Can you work these out from the drawing? Everything is in mm from the part's minimum corner. A direction names the side the tool comes from. Round coordinates to 2 decimals unless told otherwise and drop trailing zeros. Order: outer loops, then holes, each group sorted by start corner. A loop starts at its lowest first (then second) coordinate and runs counter-clockwise, first axis right, second up. Notation, with made-up numbers: (1.5, -35.5) -> (40.5, -35.5) arc R21 cw to (40.5, 3.5) -> close; hole circle Ø3 at (20.5, -5). An arc over 180 degrees is marked (long way). Use a Markdown table: item, result. Add a question column.
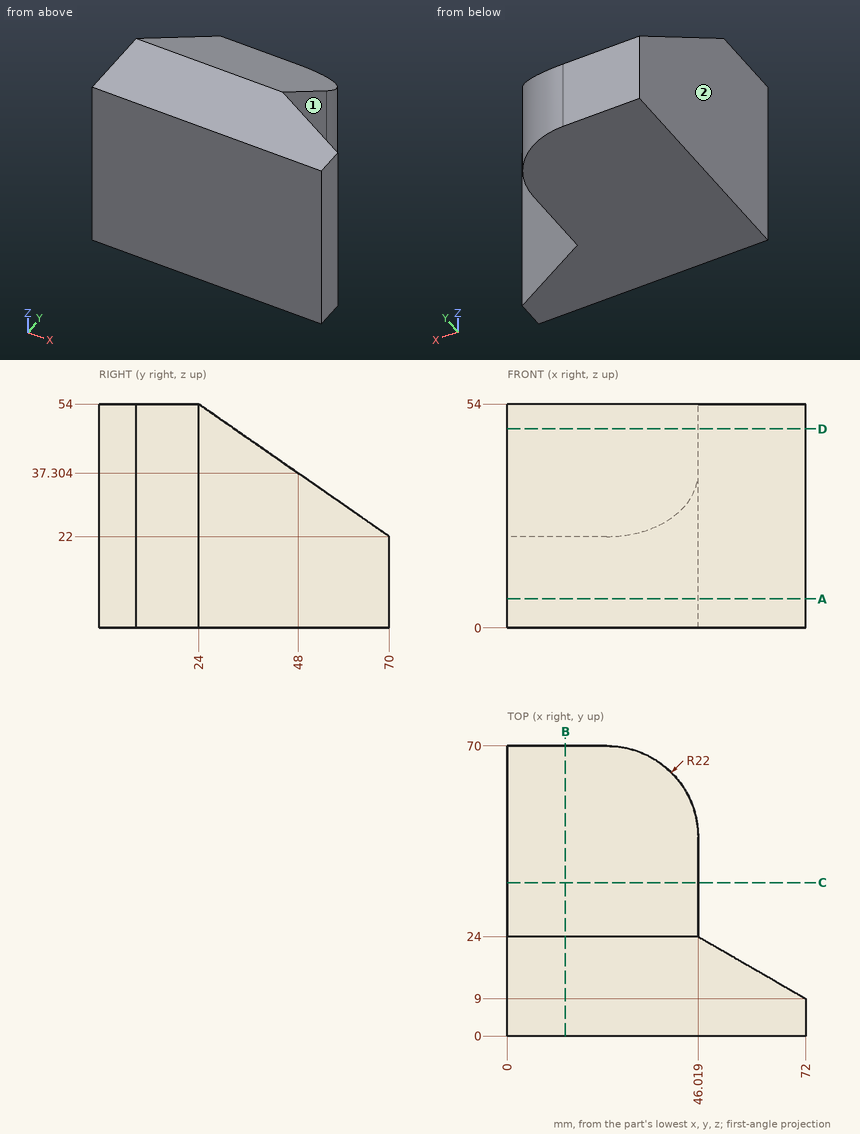
(1) I'm going to push flat-ended pins straight in: P1, Ø12, axis at y = 39, z = 31.5, coming from the +X side; P2, Ø1.5, axis at y = 15.5, z = 20, coming from the +X side; P3, Ø6, axis at x = 16, z = 30.5, coming from the +Y side (1 decimal). Where does each tip first touch, or does it pass through?
(2) Please list where these lines run through material, in increasing order: probe 1 along X at (y, z) = (39.5, 24.5); probe 2 along Z at (x, y) = (45, 32) (1 decimal); probe 3 along Z at (x, y) = (6, 29). Write a range as from..to.
(3) I want a section at A-A on z = 7. List the corners of the cut face in (x, y) for me, and give its area (3 significant figures).
(4) I want a section at C-C on y = 37. List the corners of the cut face in (x, z) for me.
(5) On a 3-axis mill with a long thin cutter (end or side, diameter ignored), from which of +Z, -Z, +X, -X, +Y, -Y can I reach the whole of each face in a straight line? I mean the marked faces 1 and 2. Say none if no direction works.
(6) I want a section at B-B on x = 14. List the corners of the cut face in (y, z) for me.
(7) I want a section at D-D on z = 48. List the corners of the cut face in (x, y) for me (1 decimal).
Output:
| question | item | result |
|---|---|---|
| 1 | P1 | x = 46.02 |
| 1 | P2 | x = 62.04 |
| 1 | P3 | y = 62.1 |
| 2 | probe 1 | 0..46.02 |
| 2 | probe 2 | 0..48.4 |
| 2 | probe 3 | 0..50.52 |
| 3 | outline | (0, 0) -> (72, 0) -> (72, 9) -> (46.02, 24) -> (46.02, 48) arc R22 ccw to (24.02, 70) -> (0, 70) -> close |
| 3 | area | 3,550 mm² |
| 4 | outline | (0, 0) -> (46.02, 0) -> (46.02, 44.96) -> (0, 44.96) -> close |
| 5 | face 1 | +Z, -Z, +X, +Y |
| 5 | face 2 | +Z, -Z, -X, +Y, -Y |
| 6 | outline | (0, 0) -> (70, 0) -> (70, 22) -> (24, 54) -> (0, 54) -> close |
| 7 | outline | (0, 0) -> (72, 0) -> (72, 9) -> (46, 24) -> (46, 32.6) -> (0, 32.6) -> close |
